Can you work these out from the model? Positions are in its coordinate system, mm. A direction names the side the tool comes from. Round coordinates to 2 decimals unless told otherwise and drop trailing zeros. Loops run counter-clockwise (first coordinate to the right, second up) from the corner with the lowest first, then second, coordinate; pieces in that order, holes last. Notation, with made-up numbers: M 87.5,-9.5 L 107.5,-9.5 A29 cw 107.5,20.5 Z; hole C 81,53.25 d7. An arc over 180 degrees is marked long. Return JSON: item names as keys, results as strings.
```python
from build123d import *

# Parameters (mm, degrees)
F0_R     = 1
F1_DEPTH = 2
F2_R     = 1
F3_DEPTH = 15
F4_DEPTH = 10
F5_DEPTH = 2


with BuildPart() as f1:
    # F0 (on Front) → F1 (new body)
    with BuildSketch(Plane.XZ):
        Polygon((-2, 1.1547005384), (-2, -1.1547005384), (0, -2.3094010768), (2, -1.1547005384), (2, 1.1547005384), (0, 2.3094010768), align=None)
        Circle(F0_R, mode=Mode.SUBTRACT)
        Circle(F0_R)
    extrude(amount=F1_DEPTH)

    # F2 (on face) → F3 (join)
    with BuildSketch(Plane(origin=(0, 0, 0), x_dir=(-1, 0, 0), z_dir=(0, 1, 0))):
        Circle(F2_R)
    extrude(amount=F3_DEPTH)

    # F2 (on face) → F4 (join)
    with BuildSketch(Plane(origin=(0, 0, 0), x_dir=(-1, 0, 0), z_dir=(0, 1, 0))):
        Circle(F2_R)
    extrude(amount=F4_DEPTH)

    # F0 (on Front) → F5 (join)
    with BuildSketch(Plane.XZ):
        Polygon((-2, 1.1547005384), (-2, -1.1547005384), (0, -2.3094010768), (2, -1.1547005384), (2, 1.1547005384), (0, 2.3094010768), align=None)
        Circle(F0_R, mode=Mode.SUBTRACT)
    extrude(amount=F5_DEPTH)


solid = f1.part
```
Q1. If I drill on line 1 along Y through (x, z) = (0.75, 1.8); line 2 along X through (y, z) = (3, 0); line 3 along Z through (x, y) = (0.3, 5), over which ranges is the centre line in solid material (lowest first)?
Results:
{"line 1": "y = -2 to 0", "line 2": "x = -1 to 1", "line 3": "z = -0.95 to 0.95"}
Q2. On a 3-axis mill with a long thin cutter (end or side, diameter ignored), from which of +Z, -Z, +X, -X, +Y, -Y can I reach the whole of each face in a straight line? I mean faces 1 (the flat face through (-1.014, -0.986, -1.724)), 2 (the cylindrical face through (0, 7, -1)). Say none if no direction works.
Results:
{"face 1": "-Z, -X, +Y, -Y", "face 2": "+Y"}
Q3. Suppose I cut it at C-C, the plane y = 7. Please give me the cut outline in (x, z), plus the area to 3 significant figures.
Results:
{"outline": "C 0,0 d2", "area": "3.14 mm2"}
Q4. Suppose I cut it at B-B, the plane x = -0.6. Please give me the cut outline in (y, z), plus the area to 3 significant figures.
Results:
{"outline": "M -2,-1.96 L 0,-1.96 L 0,-0.8 L 15,-0.8 L 15,0.8 L 0,0.8 L 0,1.96 L -2,1.96 Z", "area": "31.9 mm2"}
Q5. Suppose I cut it at A-A, the plane z = 0. Please give me the cut outline in (x, y).
Results:
{"outline": "M -2,-2 L 2,-2 L 2,0 L 1,0 L 1,15 L -1,15 L -1,0 L -2,0 Z"}
Q6. Suppose I cut it at D-D, the plane x = 1.35. Please give me the cut outline in (y, z), plus the area to 3 significant figures.
Results:
{"outline": "M -2,-1.53 L 0,-1.53 L 0,1.53 L -2,1.53 Z", "area": "6.12 mm2"}
